```python
from build123d import *

# Parameters (mm, degrees)
EXTRUDE_1_DEPTH             = 11.5
FILLET_1_R                  = 0.3
FILLET_2_R                  = 2
HOLE_WIZARD_M83_D           = 6.8
HOLE_WIZARD_M83_CSINK_D     = 8.05
HOLE_WIZARD_M83_CSINK_ANGLE = 90


with BuildPart() as part:
    # Эскиз1 → Бобышка-Вытянуть1 (new body, symmetric)
    with BuildSketch(Plane.XY):
        with BuildLine():
            Line((-5, 0), (5, 0))
            Line((5, 0), (5, -0.8))
            Line((5, -0.8), (8, -0.8))
            Line((8, -0.8), (8, -1.6))
            ThreePointArc((8, -1.6), (5.309398779, -5.576969864), (1.5, -8.5))
            Line((1.5, -8.5), (-1.5, -8.5))
            ThreePointArc((-1.5, -8.5), (-5.309398779, -5.576969864), (-8, -1.6))
            Line((-8, -1.6), (-8, -0.8))
            Line((-8, -0.8), (-5, -0.8))
            Line((-5, -0.8), (-5, 0))
        make_face()
    extrude(amount=EXTRUDE_1_DEPTH, both=True)

    # Скругление1
    fillet_1_edges = [part.edges().sort_by_distance(p)[0] for p in [
        (8, -0.8, 0),
        (8, -1.6, 0),
        (-8, -1.6, 0),
        (-8, -0.8, 0),
        (-5, 0, 0),
        (5, 0, 0),
    ]]
    fillet(fillet_1_edges, radius=FILLET_1_R)

    # Скругление2
    fillet_2_edges = [part.edges().sort_by_distance(p)[0] for p in [
        (1.5, -8.5, 0),
        (-1.5, -8.5, 0),
    ]]
    fillet(fillet_2_edges, radius=FILLET_2_R)

    # Отверстие обработанное метчиком M83 (through all)
    with Locations(Plane(origin=(0, 0, 0), x_dir=(1, 0, 0), z_dir=(0, 1, 0))):
        with Locations((0, -4.5)):
            CounterSinkHole(HOLE_WIZARD_M83_D / 2, HOLE_WIZARD_M83_CSINK_D / 2, counter_sink_angle=HOLE_WIZARD_M83_CSINK_ANGLE)

    # Эскиз5 → Повернуть1 (revolve)
    with BuildSketch(Plane(origin=(0, 0, 0), x_dir=(0, 0, -1), z_dir=(1, 0, 0))):
        with BuildLine():
            Line((6.5, -4.3), (6.5, -9.3))
            ThreePointArc((6.5, -9.3), (4, -6.8), (6.5, -4.3))
        make_face()
    revolve(axis=Axis((0, -4.3, -6.5), (0, -1, 0)))


solid = part.part
```
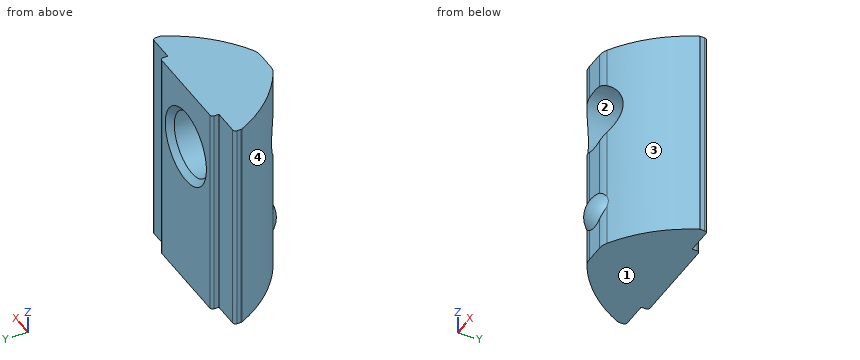
Verification items for the finished model (mm, model axes). Face numbers are marked on the shaded views. Give positions to 0.01 mm unless a question says otherwise; leave off trailing zeros. Order: outer loops, then holes, each group sorted by start corner. A loop starts at its lowest first (then second) coordinate and runs counter-clockwise, first axis right, second up. Notation, with made-up numbers: M 88.25,-4 L 95.25,-4 A25 cw 95.25,34 Z; hole C 48.5,-39.75 d7. An arc over 180 degrees is marked long. Return JSON: item names as keys, results as strings. Group by question number.
1) Mould release check, pull along X, two halves, no side actions. Record for the marked faces 1, 2, 3 and 4: pulls with the +X half, pulls with the -X half, needs draft (parallel to the pull), parting line crosses it, or undercut.
2) Section check C-C on y = -4.75. Record the cut outline in (x, z).
3) Go/stop test with flat-tipped pins: pin 1 Ø0.8 at (x, z) = (6.5, 0.5) entering from +Y; pin 2 Ø1.5 at (y, z) = (-5, 3.5) entering from -X; pin 3 Ø0.6 at (x, z) = (-0.5, 9.5) entering from -Y. Record where each tip stops, or that it passes through.
4) Scan lines: line 1 (Z direction, x = 0, y = -2.75); line 2 (X direction, y = -4, z = 1.5); line 3 (Z direction, x = 1, y = -6). Record each from-to range of solid material in increasing order.
5) Section check A-A on x = 0. Record the cut outline in (y, z) (3 decimals).
6) Section check B-B on z = -2.25. Record the cut outline in (x, y).
Answer block:
{
 "1": {"face 1": "needs draft", "face 2": "undercut", "face 3": "pulls with the +X half", "face 4": "pulls with the -X half"},
 "2": {"outline": "M -6.03,-11.5 L 6.03,-11.5 L 6.03,11.5 L -6.03,11.5 Z; hole C 0,4.5 d6.8"},
 "3": {"pin 1": "stops at y = -0.8", "pin 2": "stops at x = -6.42", "pin 3": "stops at y = -8.5"},
 "4": {"line 1": "z = -11.5 to 1.1, 7.9 to 11.5", "line 2": "x = -6.6 to -1.6, 1.6 to 6.6", "line 3": "z = -11.5 to 1.25, 7.75 to 11.5"},
 "5": {"outline": "M -8.5,-11.5 L 0,-11.5 L 0,0.475 L -0.625,1.1 L -8.5,1.1 L -8.5,-4.667 A2.5 ccw -8.5,-8.333 Z; M -8.5,7.9 L -0.625,7.9 L 0,8.525 L 0,11.5 L -8.5,11.5 Z"},
 "6": {"outline": "M -8,-1.53 A0.3 ccw -7.97,-1.66 A15 ccw -1.99,-8.22 A2 ccw -0.98,-8.5 L 0.98,-8.5 A2 ccw 1.99,-8.22 A15 ccw 7.97,-1.66 A0.3 ccw 8,-1.53 L 8,-1.1 A0.3 ccw 7.7,-0.8 L 5,-0.8 L 5,-0.3 A0.3 ccw 4.7,0 L -4.7,0 A0.3 ccw -5,-0.3 L -5,-0.8 L -7.7,-0.8 A0.3 ccw -8,-1.1 Z"}
}
